from build123d import *

# Parameters (mm, degrees)
SKETCH1_W           = 20
SKETCH1_H           = 20
BOSS_EXTRUDE1_DEPTH = 10
SKETCH4_W           = 4
SKETCH4_H           = 20
BOSS_EXTRUDE2_DEPTH = 10
BOSS_EXTRUDE3_DEPTH = 4
BOSS_EXTRUDE4_START = -4
BOSS_EXTRUDE4_DEPTH = 4
SKETCH7_R           = 0.85
CUT_EXTRUDE1_DEPTH  = 31
FILLET1_R           = 4
SKETCH8_W           = 4
SKETCH8_H           = 20
BOSS_EXTRUDE5_DEPTH = 10
SKETCH9_R           = 10
BOSS_EXTRUDE6_DEPTH = 4
BOSS_EXTRUDE7_START = -4
SKETCH10_R          = 10
BOSS_EXTRUDE7_DEPTH = 4
SKETCH12_R          = 1.1
CUT_EXTRUDE2_DEPTH  = 36.440090293
SKETCH13_R          = 6
BOSS_EXTRUDE8_DEPTH = 4
SKETCH14_R          = 1.1
CUT_EXTRUDE3_DEPTH  = 4
FILLET2_R           = 2
CUT_EXTRUDE4_REACH  = 35.166
SKETCH16_R          = 0.5


with BuildPart() as part:
    # Sketch1 → Boss-Extrude1 (new body)
    with BuildSketch(Plane(origin=(0, 0, 0), x_dir=(1, 0, 0), z_dir=(0, 1, 0))):
        Rectangle(SKETCH1_W, SKETCH1_H)
    extrude(amount=BOSS_EXTRUDE1_DEPTH)

    # Sketch4 → Boss-Extrude2 (add)
    with BuildSketch(Plane.XZ):
        with Locations((-8, 0)):
            Rectangle(SKETCH4_W, SKETCH4_H)
        with Locations((8, 0)):
            Rectangle(SKETCH4_W, SKETCH4_H)
    extrude(amount=BOSS_EXTRUDE2_DEPTH)

    # Sketch5 → Boss-Extrude3 (add)
    with BuildSketch(Plane.ZY.offset(10)):
        with BuildLine():
            Line((0, -20), (10, -20))
            Line((10, -20), (10, -10))
            ThreePointArc((10, -10), (-7.071067812, -2.928932188), (0, -20))
        make_face()
    extrude(amount=-BOSS_EXTRUDE3_DEPTH)

    # Sketch6 → Boss-Extrude4 (add)
    with BuildSketch(Plane(origin=(10, 0, 0), x_dir=(0, 0, -1), z_dir=(1, 0, 0)).offset(BOSS_EXTRUDE4_START)):
        with BuildLine():
            Line((0, -20), (-10, -20))
            Line((-10, -20), (-10, -10))
            ThreePointArc((-10, -10), (7.071067812, -2.928932188), (0, -20))
        make_face()
    extrude(amount=BOSS_EXTRUDE4_DEPTH)

    # Sketch7 → Cut-Extrude1 (cut, through all)
    with BuildSketch(Plane.ZY.offset(10)):
        with Locations((0, -10)):
            Circle(SKETCH7_R)
    extrude(amount=-CUT_EXTRUDE1_DEPTH, mode=Mode.SUBTRACT)

    # Fillet1
    fillet1_edges = [part.edges().sort_by_distance(p)[0] for p in [
        (-10, -5, 10),
        (-10, -17.071067812, -7.071067812),
        (10, -5, 10),
        (10, -17.071067812, -7.071067812),
        (-10, 0, -10),
        (10, 0, -10),
        (10, -20, 5),
        (-10, -20, 5),
    ]]
    fillet(fillet1_edges, radius=FILLET1_R - 0.0001)  # a hair under: the kernel refuses the full size

    # Sketch8 → Boss-Extrude5 (add)
    with BuildSketch(Plane(origin=(0, 10, 0), x_dir=(1, 0, 0), z_dir=(0, 1, 0))):
        with Locations((4, 0)):
            Rectangle(SKETCH8_W, SKETCH8_H)
        with Locations((-4, 0)):
            Rectangle(SKETCH8_W, SKETCH8_H)
    extrude(amount=BOSS_EXTRUDE5_DEPTH)

    # Sketch9 → Boss-Extrude6 (add)
    with BuildSketch(Plane(origin=(6, 0, 0), x_dir=(0, 0, -1), z_dir=(1, 0, 0))):
        with Locations((0, 20)):
            Circle(SKETCH9_R)
    extrude(amount=-BOSS_EXTRUDE6_DEPTH)

    # Sketch10 → Boss-Extrude7 (add)
    with BuildSketch(Plane.ZY.offset(6).offset(BOSS_EXTRUDE7_START)):
        with Locations((0, 20)):
            Circle(SKETCH10_R)
    extrude(amount=BOSS_EXTRUDE7_DEPTH)

    # Sketch12 → Cut-Extrude2 (cut, through all)
    with BuildSketch(Plane.ZY.offset(6)):
        with Locations((0, 20)):
            Circle(SKETCH12_R)
    extrude(amount=-CUT_EXTRUDE2_DEPTH, mode=Mode.SUBTRACT)

    # Sketch13 → Boss-Extrude8 (add)
    with BuildSketch(Plane(origin=(-2, 0, 0), x_dir=(0, 0, -1), z_dir=(1, 0, 0))):
        with Locations(Location((0, 20, 0), (0, 0, 180))):
            Circle(SKETCH13_R)
    extrude(amount=BOSS_EXTRUDE8_DEPTH)

    # Sketch14 → Cut-Extrude3 (cut)
    with BuildSketch(Plane(origin=(-2, 0, 0), x_dir=(0, 0, -1), z_dir=(1, 0, 0))):
        with Locations(Location((0, 20, 0), (0, 0, 180))):
            Circle(SKETCH14_R)
    extrude(amount=CUT_EXTRUDE3_DEPTH, mode=Mode.SUBTRACT)

    # Fillet2
    fillet2_edges = [part.edges().sort_by_distance(p)[0] for p in [
        (-2, 20, -6),
        (2, 20, -6),
    ]]
    fillet(fillet2_edges, radius=FILLET2_R - 0.0001)  # a hair under: the kernel refuses the full size

    # Sketch16 → Cut-Extrude4 (cut, up to next)
    with BuildSketch(Plane.XZ, mode=Mode.PRIVATE) as cut_extrude4_sk1:
        with Locations(Location((0, -6, 0), (0, 0, 270))):
            Circle(SKETCH16_R)
    cut_extrude4_tool1 = extrude(cut_extrude4_sk1.sketch, amount=-CUT_EXTRUDE4_REACH, mode=Mode.PRIVATE) & part.part
    # Sketch16 → Cut-Extrude4 (cut, up to next)
    with BuildSketch(Plane.XZ, mode=Mode.PRIVATE) as cut_extrude4_sk2:
        with Locations(Location((0, 6, 0), (0, 0, 90))):
            Circle(SKETCH16_R)
    cut_extrude4_tool2 = extrude(cut_extrude4_sk2.sketch, amount=-CUT_EXTRUDE4_REACH, mode=Mode.PRIVATE) & part.part
    add(cut_extrude4_tool1.solids().sort_by_distance((0, 0, -6))[0], mode=Mode.SUBTRACT)
    add(cut_extrude4_tool2.solids().sort_by_distance((0, 0, 6))[0], mode=Mode.SUBTRACT)


solid = part.part
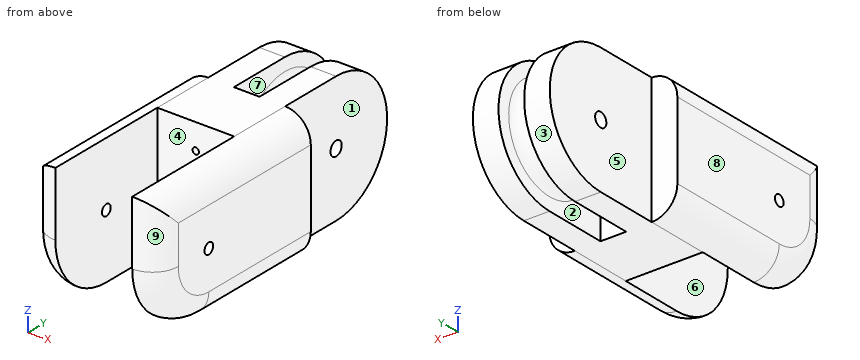
The listing builds one solid part. Answer for the finished solid, in the listing's coordinates (mm). Face numbers are marked on the shaded views. A direction names the side the tool comes from. Give positions to 0.01 mm unless a question says otherwise; leave off trailing zeros. Loops run counter-clockwise (first coordinate to the right, second up) from the corner with the lowest first, then second, coordinate; pieces in that order, holes last. Notation, with made-up numbers: (-26.5, 32.25) - (21.5, 32.25) arc R12 cw to (21.5, 37.25) - close; hole circle Ø9 at (47.25, -36). An arc over 180 degrees is marked (long way). Use one line per item in the form item = value.
1. Section C-C on y = 9 is taken. Give the vertices of the cut face in (x, z), then the cut area to 3 significant figures.
Calculated:
outline = (-10, -6) arc R4 ccw to (-6, -10) - (6, -10) arc R4 ccw to (10, -6) - (10, 6) arc R4 ccw to (6, 10) - (-6, 10) arc R4 ccw to (-10, 6) - close; hole circle Ø1 at (0, -6); hole circle Ø1 at (0, 6)
area = 385 mm^2
2. Find the intervals of material crossed by line 1 along X through (y, z) = (-9.5, 4.5); line 2 along X through (y, z) = (24.5, -6.5); line 3 along Z through (x, y) = (6.25, 0), in increasing order. Write a range as [from, to].
Calculated:
line_1 = [-10, -6], [6, 10]
line_2 = [-6, -2], [2, 6]
line_3 = [-9.99, 9.99]
3. The mould has two halves that part along X. Classify the marked faces 6, 7, 8 and 9: pulls with the +X half, pulls with the -X half, needs draft (parallel to the pull), parting line crosses it, or undercut.
Calculated:
face_6 = undercut
face_7 = undercut
face_8 = pulls with the -X half
face_9 = pulls with the +X half
4. Which of the six approach directions +Z, -Z, +X, -X, +Y, -Y give full straight-line access (tool end or side, diameter ignored) to the marked faces 1, 2, 3, 4 and 5?
Calculated:
face_1 = +Z, -Z, +X, +Y
face_2 = none
face_3 = +X, -X, +Y
face_4 = +Z, -Z, -Y
face_5 = +Z, -Z, -X, +Y
5. Given pin 1 Ø1.5 at (x, z) = (6, -4.5) entering from -Y; pin 2 Ø10 at (y, z) = (21.5, 1) entering from +X; pin 3 Ø1.2 at (x, z) = (-7.5, 0) entering from +Y, each flat-ended and moving along its own axis, determine where each tip first touches the part or whether it passes through.
Calculated:
pin_1 = -19.27
pin_2 = 6
pin_3 = 10
6. Section B-B on x = 4.5 is taken. Give the vertices of the cut face in (y, z).
Calculated:
outline = (0, -10) - (20, -10) arc R10 ccw to (20, 10) - (0, 10) - close; hole circle Ø2.2 at (20, 0)
7. Section D-D on x = -7 is taken. Give the vertices of the cut face in (y, z), then the cut area to 3 significant figures.
Calculated:
outline = (-19.87, 0) arc R9.87 ccw to (-10, -9.87) - (10, -9.87) - (10, 9.87) - (-19.87, 9.87) - close; hole circle Ø1.7 at (-10, 0)
area = 567 mm^2
